Here's how the part is built. I have some questions about the finished solid (model axes, mm). A direction names the side the tool comes from. Coordinates: 2 decimals unless noted, no trailing zeros. Write each loop counter-clockwise with the first axis right and the second up, starting at its lowest first coordinate (ties: lowest second). Pieces come first, ordered by that corner, then holes.
Item 1: We'd pull the mould along Z, two halves only. Please class faces 6 (the face through (48, 14.6, 71)), 7 (the face through (48, 16, 75.6)), 8 (the face through (46, 16, 70)): +Z half, -Z half, draft (parallel to the pull), parting line (faces both ways), or undercut.
Item 2: If we section it at C-C (x = 42): Please give me the cut outline in (y, z), then the cut area to 3 significant figures.
Item 3: If we section it at D-D (x = 51): Please give me the cut outline in (y, z).
Item 4: If we section it at B-B (y = 0): Please give me the cut outline in (x, z), then the cut area to 3 significant figures.
Item 5: If I drill on line 1 (X direction, y = -0.5, z = 63.5); line 2 (Y direction, x = 44.5, z = 67.5); line 3 (Z direction, x = 59, y = 10.5), over which ranges is the centre line in solid material (lowest first)?
Item 6: I'm going to push flat-ended pins straight in: pin 1 Ø6.5 at (x, z) = (49.5, 68) entering from +Y; pin 2 Ø1 at (y, z) = (16.5, 69.5) entering from -X; pin 3 Ø5 at (x, z) = (45.5, 66.5) entering from +Y; pin 4 Ø4 at (x, z) = (54.5, 67.5) entering from +Y. Where does each tip first touch, or does it pass through?
Item 7: If we section it at A-A (z = 69.25): Please give me the cut outline in (x, y), then the cut area to 3 significant figures.
Item 8: For faces 1 (the face through (50.86, -8.1, 63.18)), 2 (the face through (52, 16, 70)), 3 (the face through (50, 16, 70)), 4 (the face through (48, 17.4, 71)), 5 (the face through (44, 16, 70)), which set-ups out of +Z, -Z, +X, -X, +Y, -Y let a thin tool reach every point of the face, with its end or its side?
from build123d import *

# Parameters (mm, degrees)
SKETCH1_R                        = 18.6
CAP_DISC_DEPTH                   = 2.8
SKETCH2_W                        = 8
SKETCH2_H                        = 2.8
STRAIN_RELIEF_TAB_DEPTH          = 11
PH_ELECTRODE_BORE_DEPTH          = 71.512126617
PH_ELECTRODE_BORE_DEPTH_BACK     = 71.512126617
SKETCH3_R                        = 6.3
CABLE_AND_HOSE_WINDOW_DEPTH      = 71.512126617
CABLE_AND_HOSE_WINDOW_DEPTH_BACK = 71.512126617
ZIP_TIE_SLOT_DEPTH               = 106.59109811
ZIP_TIE_SLOT_DEPTH_BACK          = 106.59109811
SKETCH5_W                        = 4
SKETCH5_H                        = 2


with BuildPart() as part:
    # Sketch1 → Cap_disc (new body)
    with BuildSketch(Plane.XY.offset(61.8)):
        with Locations((48, 0)):
            Circle(SKETCH1_R)
    extrude(amount=CAP_DISC_DEPTH)

    # Sketch2 → Strain_relief_tab (add)
    with BuildSketch(Plane.XY.offset(64.6)):
        with Locations((48, 16)):
            Rectangle(SKETCH2_W, SKETCH2_H)
    extrude(amount=STRAIN_RELIEF_TAB_DEPTH)

    # Sketch3 → pH_electrode_bore (cut, two sides: drawn at the far end of the back side and taken through both)
    with BuildSketch(Plane.XY.offset(61.8).offset(-PH_ELECTRODE_BORE_DEPTH_BACK)):
        with Locations((42, 0)):
            Circle(SKETCH3_R)
    extrude(amount=PH_ELECTRODE_BORE_DEPTH + PH_ELECTRODE_BORE_DEPTH_BACK, mode=Mode.SUBTRACT)

    # Sketch4 → Cable_and_hose_window (cut, two sides: drawn at the far end of the back side and taken through both)
    with BuildSketch(Plane.XY.offset(61.8).offset(-CABLE_AND_HOSE_WINDOW_DEPTH_BACK)):
        with BuildLine():
            Line((53, -9), (58, -9))
            ThreePointArc((58, -9), (60.121320344, -8.121320344), (61, -6))
            Line((61, -6), (61, 6))
            ThreePointArc((61, 6), (60.121320344, 8.121320344), (58, 9))
            Line((58, 9), (53, 9))
            ThreePointArc((53, 9), (50.878679656, 8.121320344), (50, 6))
            Line((50, 6), (50, -6))
            ThreePointArc((50, -6), (50.878679656, -8.121320344), (53, -9))
        make_face()
    extrude(amount=CABLE_AND_HOSE_WINDOW_DEPTH + CABLE_AND_HOSE_WINDOW_DEPTH_BACK, mode=Mode.SUBTRACT)

    # Sketch5 → Zip_tie_slot (cut, two sides: drawn at the far end of the back side and taken through both)
    with BuildSketch(Plane(origin=(0, 13, 0), x_dir=(1, 0, 0), z_dir=(0, 1, 0)).offset(-ZIP_TIE_SLOT_DEPTH_BACK)):
        with Locations((48, -69.6)):
            Rectangle(SKETCH5_W, SKETCH5_H)
    extrude(amount=ZIP_TIE_SLOT_DEPTH + ZIP_TIE_SLOT_DEPTH_BACK, mode=Mode.SUBTRACT)


solid = part.part
Answer list:
1. face 6: draft
1. face 7: +Z half
1. face 8: undercut
2. outline: (-17.61, 61.8) - (-6.3, 61.8) - (-6.3, 64.6) - (-17.61, 64.6) - close; (6.3, 61.8) - (17.61, 61.8) - (17.61, 64.6) - (6.3, 64.6) - close
2. area: 63.3 mm2
3. outline: (-18.36, 61.8) - (-8.24, 61.8) - (-8.24, 64.6) - (-18.36, 64.6) - close; (8.24, 61.8) - (18.36, 61.8) - (18.36, 64.6) - (17.4, 64.6) - (17.4, 75.6) - (14.6, 75.6) - (14.6, 64.6) - (8.24, 64.6) - close
4. outline: (29.4, 61.8) - (35.7, 61.8) - (35.7, 64.6) - (29.4, 64.6) - close; (48.3, 61.8) - (50, 61.8) - (50, 64.6) - (48.3, 64.6) - close; (61, 61.8) - (66.6, 61.8) - (66.6, 64.6) - (61, 64.6) - close
4. area: 38.1 mm2
5. line 1: x = 29.41 to 35.72, 48.28 to 50, 61 to 66.59
5. line 2: y = 14.6 to 17.4
5. line 3: z = 61.8 to 64.6
6. pin 1: stops at y = 17.4
6. pin 2: stops at x = 44
6. pin 3: stops at y = 18.58
6. pin 4: passes through
7. outline: (44, 14.6) - (46, 14.6) - (46, 17.4) - (44, 17.4) - close; (50, 14.6) - (52, 14.6) - (52, 17.4) - (50, 17.4) - close
7. area: 11.2 mm2
8. face 1: +Z, -Z
8. face 2: +Z, +X, +Y, -Y
8. face 3: +Y, -Y
8. face 4: +Z, +X, -X, +Y
8. face 5: +Z, -X, +Y, -Y
